```python
from build123d import *

# Parameters (mm, degrees)
F0_W     = 45.323744
F0_H     = 27.477518
F1_DEPTH = 25
F2_R     = 3.125
F3_DEPTH = 50


with BuildPart() as f1:
    # F0 (on Front) → F1 (new body)
    with BuildSketch(Plane.XZ):
        with Locations((-13.172213, 13.738759)):
            Rectangle(F0_W, F0_H)
    extrude(amount=F1_DEPTH)

    # F2 (on face) → F3 (cut, symmetric)
    with BuildSketch(Plane.YZ.offset(9.489659)):
        with Locations((-13.99685, 13.850922)):
            Circle(F2_R)
    extrude(amount=F3_DEPTH, both=True, mode=Mode.SUBTRACT)


solid = f1.part
```
Input: part model. Units: mm. Frame: model coordinates. Round coordinates to 2 decimals unless told otherwise and drop trailing zeros. Order: outer loops, then holes, each group sorted by start corner. A loop starts at its lowest first (then second) coordinate and runs counter-clockwise, first axis right, second up. Notation, with made-up numbers: (14.5, -35) - (52.5, -35) arc R26 ccw to (52.5, -19) - close; hole circle Ø11 at (-14.5, 86.5). An arc over 180 degrees is marked (long way). One line per question, with ' | ' between items. Start each with the question number.
1) Cut plane A-A, the plane z = 15. Return the cut outline in (x, y).
2) Cut plane C-C, the plane x = -1. Return the cut outline in (y, z) (3 decimals), then the cut area to 3 significant figures.
3) Ray query, probe 1 along Y at (x, z) = (6, 14.75); probe 2 along Z at (x, y) = (4, -15); probe 3 along Y at (x, z) = (-3, 13.5). Return the intervals inside material, ascending.
4) Contact query for a flat-ended pin moving along its axis: P1, Ø1, axis at x = -7.5, y = -8.5, coming from the -Z side. Output: stop coordinate, or through.
5) Cut plane B-B, the plane y = -13.75. Return the cut outline in (x, z), then the cut area to 3 significant figures.
6) Pull-direction query (Z, two-part tool) for faces 1 (the cylindrical face through (-12.855, -16.477, 11.949)), 2 (the flat face through (-13, -12, 27.478)), 3 (the flat face through (-13, -12, 0)), 4 (the flat face through (-13, 0, 14)); classes: +Z half, -Z half, draft (parallel to the pull), parting line (faces both ways), or undercut.
Worked out:
1) outline: (-35.83, -25) - (9.49, -25) - (9.49, -16.9) - (-35.83, -16.9) - close; (-35.83, -11.09) - (9.49, -11.09) - (9.49, 0) - (-35.83, 0) - close
2) outline: (-25, 0) - (0, 0) - (0, 27.478) - (-25, 27.478) - close; hole circle Ø6.25 at (-13.997, 13.851) | area: 656 mm^2
3) probe 1: y = -25 to -16.99, -11 to 0 | probe 2: z = 0 to 10.89, 16.81 to 27.48 | probe 3: y = -25 to -17.1, -10.89 to 0
4) P1: stops at z = 0
5) outline: (-35.83, 0) - (9.49, 0) - (9.49, 10.74) - (-35.83, 10.74) - close; (-35.83, 16.97) - (9.49, 16.97) - (9.49, 27.48) - (-35.83, 27.48) - close | area: 963 mm^2
6) face 1: undercut | face 2: +Z half | face 3: -Z half | face 4: draft
